```python
from build123d import *

# Parameters (mm, degrees)
SKETCH6_W               = 40
SKETCH6_H               = 2
BOSS_EXTRUDE4_DEPTH     = 16
SKETCH9_R               = 3.25
CUT_EXTRUDE2_DEPTH      = 2
CUT_EXTRUDE1_DEPTH      = 26.690465157
CUT_EXTRUDE1_DEPTH_BACK = 16
SKETCH7_W               = 42.708590122
SKETCH7_H               = 18.182038554
SKETCH12_W              = 23.999933515
SKETCH12_H              = 26
SKETCH12_R              = 1.75
BOSS_EXTRUDE8_DEPTH     = 2


with BuildPart() as part:
    # Sketch6 → Boss-Extrude4 (new body)
    with BuildSketch(Plane(origin=(0, 0, 0), x_dir=(1, 0, 0), z_dir=(0, 1, 0))):
        with Locations((0, -12)):
            Rectangle(SKETCH6_W, SKETCH6_H)
    extrude(amount=BOSS_EXTRUDE4_DEPTH)

    # Sketch9 → Cut-Extrude2 (cut)
    with BuildSketch(Plane(origin=(0, 0, 11), x_dir=(-1, 0, 0), z_dir=(0, 0, -1))):
        with Locations((-12, 8)):
            Circle(SKETCH9_R)
    extrude(amount=-CUT_EXTRUDE2_DEPTH, mode=Mode.SUBTRACT)

    # Sketch7 → Cut-Extrude1 (cut, two sides: drawn at the far end of the back side and taken through both)
    with BuildSketch(Plane(origin=(0, 0, 11), x_dir=(-1, 0, 0), z_dir=(0, 0, -1)).offset(-CUT_EXTRUDE1_DEPTH_BACK)):
        with Locations((0, 8)):
            Rectangle(SKETCH7_W, SKETCH7_H)
        with BuildLine():
            Line((-5.942038411, 16), (-12, 16))
            ThreePointArc((-12, 16), (-19.39103626, 11.061467459), (-17.656854249, 2.343145751))
            Line((-17.656854249, 2.343145751), (-15.313708499, 0))
            Line((-15.313708499, 0), (20, 0))
            Line((20, 0), (20, 1.767244224))
            ThreePointArc((20, 1.767244224), (19.761112544, 2.715127447), (19.101517394, 3.43657326))
            Line((19.101517394, 3.43657326), (5.07313553, 12.69329036))
            ThreePointArc((5.07313553, 12.69329036), (-0.191638738, 15.155492779), (-5.942038411, 16))
        make_face(mode=Mode.SUBTRACT)
    extrude(amount=CUT_EXTRUDE1_DEPTH + CUT_EXTRUDE1_DEPTH_BACK, mode=Mode.SUBTRACT)


with BuildPart() as body_2:
    # Mirror2: mirrored copy
    add(part.part.mirror(Plane.XY))


with BuildPart() as part_1:
    add(part.part)

    add(body_2.part)  # Boss-Extrude8 merges body 2
    # Sketch12 → Boss-Extrude8 (add)
    with BuildSketch(Plane(origin=(0, 0, 0), x_dir=(1, 0, 0), z_dir=(0, 1, 0))):
        with Locations((-8.000033242, 0)):
            Rectangle(SKETCH12_W, SKETCH12_H)
        with Locations(Location((-13.000047854, 0, 0), (0, 0, 270))):
            Circle(SKETCH12_R, mode=Mode.SUBTRACT)
        with Locations(Location((-3.000047854, 0, 0), (0, 0, 270))):
            Circle(SKETCH12_R, mode=Mode.SUBTRACT)
    extrude(amount=BOSS_EXTRUDE8_DEPTH)


solid = part_1.part
```
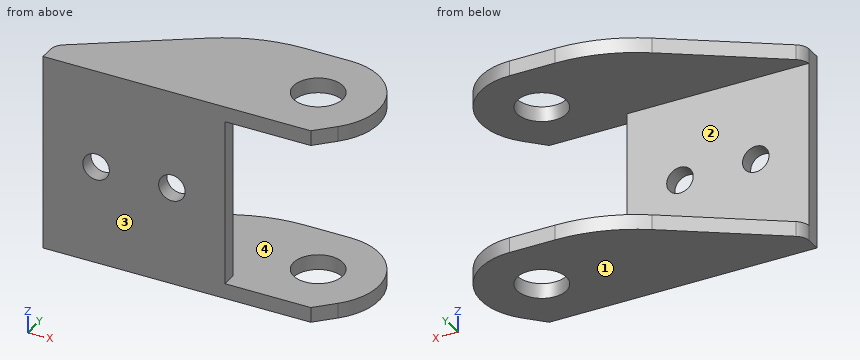
Could you check a few things on this model? Use its own coordinates, in mm. Face numbers are marked on the shaded views. Give positions to 0.01 mm unless a question says otherwise; leave off trailing zeros. Loops run counter-clockwise (first coordinate to the right, second up) from the corner with the lowest first, then second, coordinate; pieces in that order, holes last. Notation, with made-up numbers: (27, 12.25) - (53, 12.25) arc R27 cw to (53, 37.25) - close; hole circle Ø2 at (12.25, -22.75). An arc over 180 degrees is marked (long way). Use one line per item in the form item = value.
1. I want a section at B-B (x = 7.5). Please give me the cut outline in (y, z).
Response values:
outline = (0, -13) - (16, -13) - (16, -11) - (0, -11) - close; (0, 11) - (16, 11) - (16, 13) - (0, 13) - close
2. I want a section at A-A (z = 0). Please give me the cut outline in (x, y), and give its area (3 significant figures).
Response values:
outline = (-20, 0) - (-14.75, 0) - (-14.75, 2) - (-20, 2) - close; (-11.25, 0) - (-4.75, 0) - (-4.75, 2) - (-11.25, 2) - close; (-1.25, 0) - (4, 0) - (4, 2) - (-1.25, 2) - close
area = 34.0 mm²
3. I want a section at C-C (y = 12.25). Please give me the cut outline in (x, z).
Response values:
outline = (-5.74, -13) - (18.78, -13) - (18.78, -11) - (-5.74, -11) - close; (-5.74, 11) - (18.78, 11) - (18.78, 13) - (-5.74, 13) - close
4. I want a section at D-D (x = 11.5). Please give me the cut outline in (y, z).
Response values:
outline = (0, -13) - (4.79, -13) - (4.79, -11) - (0, -11) - close; (0, 11) - (4.79, 11) - (4.79, 13) - (0, 13) - close; (11.21, -13) - (16, -13) - (16, -11) - (11.21, -11) - close; (11.21, 11) - (16, 11) - (16, 13) - (11.21, 13) - close
5. Thinking about a two-plate mould opening in Z: for the marked faces 1, 2, 3 and 4, which applies, released by +Z, released by -Z, zero draft, split by the parting line, or undercut?
Response values:
face_1 = released by -Z
face_2 = undercut
face_3 = zero draft
face_4 = undercut
6. I'm going to push flat-ended pins straight in: pin 1 Ø4 at (x, y) = (-4, 13.5) entering from +Z; pin 2 Ø1 at (x, z) = (-10.5, -7.5) entering from +Y; pin 3 Ø1.6 at (y, z) = (0.5, 3) entering from +X. Where does each tip first touch, or does it pass through?
Response values:
pin_1 = 13
pin_2 = 2
pin_3 = 4
7. I need wall thicknesses on probe 1 along Z at (x, y) = (8.5, 8.25); probe 2 along X at (y, z) = (1, 0); probe 3 along Y at (x, z) = (12, 12.45). Which ranges of each line are inside material? Lowest first, please.
Response values:
probe_1 = -13 to -11, 11 to 13
probe_2 = -20 to -14.75, -11.25 to -4.75, -1.25 to 4
probe_3 = 0 to 4.75, 11.25 to 16
